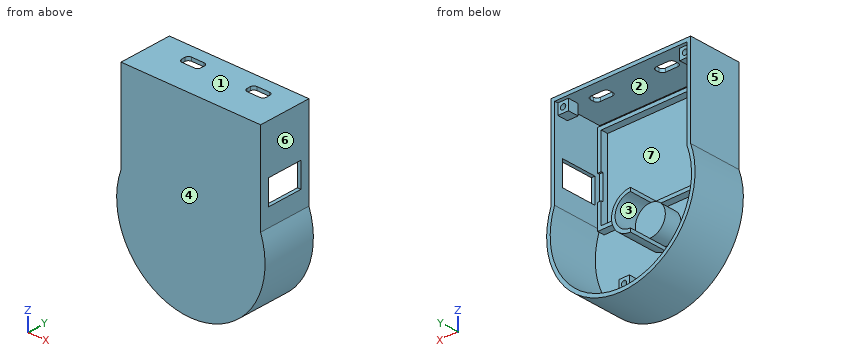
```python
from build123d import *

# Parameters (mm, degrees)
BOSS_EXTRUDE1_DEPTH = 2
BOSS_EXTRUDE2_DEPTH = 30
BOSS_EXTRUDE3_DEPTH = 22
SKETCH4_R           = 8.495
BOSS_EXTRUDE4_DEPTH = 9.7
SKETCH5_W           = 6
SKETCH5_H           = 6
SKETCH5_R           = 1.5
BOSS_EXTRUDE5_DEPTH = 26
SKETCH6_W           = 75
SKETCH6_H           = 20
CUT_EXTRUDE1_DEPTH  = 6
SKETCH8_W           = 70
SKETCH8_H           = 50
SKETCH8_W_2         = 66
SKETCH8_H_2         = 46
BOSS_EXTRUDE6_DEPTH = 4
SKETCH9_W           = 11
SKETCH9_H           = 6
CUT_EXTRUDE3_DEPTH  = 4
FILLET1_R           = 2
SKETCH10_W          = 14
SKETCH10_H          = 20
CUT_EXTRUDE4_DEPTH  = 10


with BuildPart() as part:
    # Sketch1 → Boss-Extrude1 (new body)
    with BuildSketch(Plane(origin=(0, 0, 0), x_dir=(1, 0, 0), z_dir=(0, 1, 0))):
        with BuildLine():
            Line((-37.5, 25), (-37.5, -25))
            Line((-37.5, -25), (37.5, -25))
            Line((37.5, -25), (37.5, 25))
            ThreePointArc((37.5, 25), (0, 78.919410907), (-37.5, 25))
        make_face()
    extrude(amount=BOSS_EXTRUDE1_DEPTH)

    # Sketch2 → Boss-Extrude2 (add)
    with BuildSketch(Plane.XZ):
        with BuildLine():
            Line((-39.5, -24.645308483), (-39.5, 27))
            Line((-39.5, 27), (39.5, 27))
            Line((39.5, 27), (39.5, -24.645308483))
            ThreePointArc((39.5, -24.645308483), (0, -80.919410907), (-39.5, -24.645308483))
        make_face()
        with BuildLine():
            Line((-37.5, -25), (-37.5, 25))
            Line((-37.5, 25), (37.5, 25))
            Line((37.5, 25), (37.5, -25))
            ThreePointArc((37.5, -25), (0, -78.919410907), (-37.5, -25))
        make_face(mode=Mode.SUBTRACT)
    extrude(amount=-BOSS_EXTRUDE2_DEPTH)

    # Sketch3 → Boss-Extrude3 (add)
    with BuildSketch(Plane(origin=(0, 2, 0), x_dir=(1, 0, 0), z_dir=(0, 1, 0))):
        with BuildLine():
            Line((0, 49.669410907), (0, 47.669410907))
            ThreePointArc((0, 47.669410907), (8.75, 38.919410907), (0, 30.169410907))
            Line((0, 30.169410907), (0, 28.169410907))
            ThreePointArc((0, 28.169410907), (10.75, 38.919410907), (0, 49.669410907))
        make_face()
    extrude(amount=BOSS_EXTRUDE3_DEPTH)

    # Sketch4 → Boss-Extrude4 (add)
    with BuildSketch(Plane(origin=(0, 2, 0), x_dir=(1, 0, 0), z_dir=(0, 1, 0))):
        with Locations(Location((0, 38.919410907, 0), (0, 0, 270))):
            Circle(SKETCH4_R)
    extrude(amount=BOSS_EXTRUDE4_DEPTH)

    # Sketch5 → Boss-Extrude5 (add)
    # profile 1 of 3: a face of its own
    with BuildSketch(Plane(origin=(0, 2, 0), x_dir=(1, 0, 0), z_dir=(0, 1, 0))):
        with Locations((-34.5, -22)):
            Rectangle(SKETCH5_W, SKETCH5_H)
        with Locations(Location((-34.5, -22, 0), (0, 0, 90))):
            Circle(SKETCH5_R, mode=Mode.SUBTRACT)
    # profile 2 of 3: a face of its own
    with BuildSketch(Plane(origin=(0, 2, 0), x_dir=(1, 0, 0), z_dir=(0, 1, 0))):
        with Locations((34.5, -22)):
            Rectangle(SKETCH5_W, SKETCH5_H)
        with Locations(Location((34.5, -22, 0), (0, 0, 90))):
            Circle(SKETCH5_R, mode=Mode.SUBTRACT)
    # profile 3 of 3: a face of its own
    with BuildSketch(Plane(origin=(0, 2, 0), x_dir=(1, 0, 0), z_dir=(0, 1, 0))):
        with Locations((0, 76.087024619)):
            Rectangle(SKETCH5_W, SKETCH5_H)
        with Locations(Location((0, 76.087024619, 0), (0, 0, 90))):
            Circle(SKETCH5_R, mode=Mode.SUBTRACT)
    extrude(amount=BOSS_EXTRUDE5_DEPTH)

    # Sketch6 → Cut-Extrude1 (cut)
    with BuildSketch(Plane(origin=(0, 0, 19), x_dir=(-1, 0, 0), z_dir=(0, 0, -1))):
        with Locations((0, 12)):
            Rectangle(SKETCH6_W, SKETCH6_H)
    extrude(amount=-CUT_EXTRUDE1_DEPTH, mode=Mode.SUBTRACT)

    # Sketch8 → Boss-Extrude6 (add)
    with BuildSketch(Plane(origin=(0, 2, 0), x_dir=(1, 0, 0), z_dir=(0, 1, 0))):
        with Locations((0, 3.5)):
            Rectangle(SKETCH8_W, SKETCH8_H)
        with Locations((0, 3.5)):
            Rectangle(SKETCH8_W_2, SKETCH8_H_2, mode=Mode.SUBTRACT)
    extrude(amount=BOSS_EXTRUDE6_DEPTH)

    # Sketch9 → Cut-Extrude3 (cut)
    with BuildSketch(Plane.XY.offset(27)):
        with Locations((-17, 20)):
            Rectangle(SKETCH9_W, SKETCH9_H)
        with Locations((20, 20)):
            Rectangle(SKETCH9_W, SKETCH9_H)
    extrude(amount=-CUT_EXTRUDE3_DEPTH, mode=Mode.SUBTRACT)

    # Fillet1
    fillet1_edges = [part.edges().sort_by_distance(p)[0] for p in [
        (-22.5, 17, 26),
        (-22.5, 23, 26),
        (-11.5, 23, 26),
        (-11.5, 17, 26),
        (14.5, 17, 26),
        (14.5, 23, 26),
        (25.5, 23, 26),
        (25.5, 17, 26),
    ]]
    fillet(fillet1_edges, radius=FILLET1_R)

    # Sketch10 → Cut-Extrude4 (cut)
    with BuildSketch(Plane(origin=(39.5, 0, 0), x_dir=(0, 0, -1), z_dir=(1, 0, 0))):
        with Locations((7.50936627, 15)):
            Rectangle(SKETCH10_W, SKETCH10_H)
    extrude(amount=-CUT_EXTRUDE4_DEPTH, mode=Mode.SUBTRACT)


solid = part.part
```
Geometry: final body of the model. Coordinates: model frame, mm. Face numbers are marked on the shaded views. A direction names the side the tool comes from. Round coordinates to 2 decimals unless told otherwise and drop trailing zeros. Write each loop counter-clockwise with the first axis right and the second up, starting at its lowest first coordinate (ties: lowest second). Pieces come first, ordered by that corner, then holes.
Item 1: Mould query, pull axis X, two halves, no side actions, for the marked faces 4, 5, 6 and 7. Classes: +X half, -X half, draft (parallel to the pull), parting line (faces both ways), or undercut.
Item 2: Pin query (flat end, axial travel): P1, Ø4, axis at x = 34.5, z = 22, coming from the +Y side; P2, Ø1.2, axis at x = -13, y = 5, coming from the -Z side; P3, Ø1, axis at x = 39, y = 14.5, coming from the -Z side. Return the tip coordinate at first contact, or that it passes through.
Item 3: Section query B-B (z = -3). Return loops of the section in (x, y).
Item 4: Section query D-D (z = -70). Return loops of the section in (x, y).
Item 5: Set-up query: the marked faces 1, 2 and 3. Return all of +Z, -Z, +X, -X, +Y, -Y with unobstructed straight access to the full face (end or side cutting, diameter ignored); none if empty.
Item 6: Section query A-A (y = 13). Return loops of the section in (x, z).
Item 7: Material intervals for L1, parallel to X at y = 23.4, z = 22; L2, parallel to X at y = 3, z = -17.5; L3, parallel to Y at x = -4.5, z = -54.5, sorted ascending.
Item 8: Section query C-C (z = -52). Return loops of the section in (x, y), plus the area to 3 significant figures.
Completed:
1. face 4: draft
1. face 5: -X half
1. face 6: +X half
1. face 7: undercut
2. P1: stops at y = 28
2. P2: stops at z = -79.05
2. P3: stops at z = -55.7
3. outline: (-39.5, 0) - (39.5, 0) - (39.5, 5) - (37.5, 5) - (37.5, 2) - (35, 2) - (35, 5) - (33, 5) - (33, 2) - (-33, 2) - (-33, 6) - (-35, 6) - (-35, 2) - (-37.5, 2) - (-37.5, 30) - (-39.5, 30) - close; (37.5, 25) - (39.5, 25) - (39.5, 30) - (37.5, 30) - close
4. outline: (-28.25, 0) - (28.25, 0) - (28.25, 30) - (25.18, 30) - (25.18, 2) - (-25.18, 2) - (-25.18, 30) - (-28.25, 30) - close
5. face 1: +Z, +X, -X, +Y, -Y
5. face 2: none
5. face 3: +Y
6. outline: (-39.5, -24.65) arc R42 ccw (long way) to (39.5, -24.65) - (39.5, -14.51) - (37.5, -14.51) - (37.5, -25) arc R40 cw to (3, -78.81) - (3, -73.09) - (-3, -73.09) - (-3, -78.81) arc R40 cw to (-37.5, -25) - (-37.5, 25) - (37.5, 25) - (37.5, -0.51) - (39.5, -0.51) - (39.5, 27) - (-39.5, 27) - close; (0, -49.67) arc R10.75 ccw to (0, -28.17) - (0, -30.17) arc R8.75 cw to (0, -47.67) - close; hole circle Ø3 at (0, -76.09)
7. L1: x = -39.5 to -36, -33 to -31.5, 31.5 to 33, 36 to 39.5
7. L2: x = -39.5 to -37.5, -35 to -33, 33 to 35, 37.5 to 39.5
7. L3: y = 0 to 2
8. outline: (-39.91, 0) - (39.91, 0) - (39.91, 30) - (37.8, 30) - (37.8, 2) - (-37.8, 2) - (-37.8, 30) - (-39.91, 30) - close
8. area: 278 mm2
